```python
from build123d import *

# Parameters (mm, degrees)
SKETCH1_R           = 4
SKETCH1_R_2         = 5
BOSS_EXTRUDE1_DEPTH = 8
SKETCH2_R           = 7.75
CUT_EXTRUDE1_DEPTH  = 9


with BuildPart() as part:
    # Sketch1 → Boss-Extrude1 (new body)
    with BuildSketch(Plane.XY):
        Polygon((-55.929590299, 11.283196531), (55.49624814, 11.283196531), (55.49624814, -41.637870342), (-55.929590299, -41.637870342), (-55.929590299, -36.557898132), align=None)
        with Locations((38.28332892, -7.416803469)):
            Circle(SKETCH1_R, mode=Mode.SUBTRACT)
        with Locations((-0.21667108, -10.716803469)):
            Circle(SKETCH1_R_2, mode=Mode.SUBTRACT)
        with Locations((-38.71667108, -7.416803469)):
            Circle(SKETCH1_R, mode=Mode.SUBTRACT)
    extrude(amount=BOSS_EXTRUDE1_DEPTH)

    # Sketch2 → Cut-Extrude1 (cut, through all)
    with BuildSketch(Plane.XY.offset(8)):
        with Locations((-0.21667108, -10.716803469)):
            Circle(SKETCH2_R)
    extrude(amount=-CUT_EXTRUDE1_DEPTH, mode=Mode.SUBTRACT)


solid = part.part
```
Can you work these out from the model? Positions are in its coordinate system, mm. Coordinates: 2 decimals unless noted, no trailing zeros. Loops run counter-clockwise (first coordinate to the right, second up) from the corner with the lowest first, then second, coordinate; pieces in that order, holes last. Notation, with made-up numbers: M -33,81 L 21,81 A19 cw 21,87 Z; hole C 16.5,44 d2. An arc over 180 degrees is marked long. Put each result on its own line as item: value. Start each with the question number.
(1) Will this pin go through, and if not, where does the flat tip stop? pin 1 Ø5 at (x, y) = (-3, -14) entering from +Z.
(2) We'd pull the mould along X, two halves only. Please class faces 1 (the face through (-34.9, -6.22, 3.94)), 2 (the face through (-55.93, -15, 4)), 3 (the face through (1, -41.638, 4)): +X half, -X half, draft (parallel to the pull), parting line (faces both ways), or undercut.
(3) Imagine slicing it at A-A on x = -41.5. List the corners of the cut face in (y, z) for me, and give its area (3 significant figures).
(4) Imagine slicing it at C-C on y = -15. List the corners of the cut face in (x, z) for me, and give its area (3 significant figures).
(5) Imagine slicing it at B-B on z = 2.75. List the corners of the cut face in (x, y) for me.
(6) I need wall thicknesses on probe 1 along X at (y, z) = (-5.5, 6.75); probe 2 along X at (y, z) = (-8, 2.75); probe 3 along X at (y, z) = (-17, 7.75). Which ranges of each line are inside material? Lowest first, please.
Worked answers:
1. pin 1: passes through
2. face 1: undercut
2. face 2: -X half
2. face 3: draft
3. outline: M -41.64,0 L -10.29,0 L -10.29,8 L -41.64,8 Z; M -4.54,0 L 11.28,0 L 11.28,8 L -4.54,8 Z
3. area: 377 mm2
4. outline: M -55.93,0 L -6.68,0 L -6.68,8 L -55.93,8 Z; M 6.24,0 L 55.5,0 L 55.5,8 L 6.24,8 Z
4. area: 788 mm2
5. outline: M -55.93,-41.64 L 55.5,-41.64 L 55.5,11.28 L -55.93,11.28 Z; hole C -38.72,-7.42 d8; hole C -0.22,-10.72 d15.5; hole C 38.28,-7.42 d8
6. probe 1: x = -55.93 to -42.23, -35.21 to -5.95, 5.51 to 34.77, 41.79 to 55.5
6. probe 2: x = -55.93 to -42.67, -34.76 to -7.47, 7.04 to 34.33, 42.24 to 55.5
6. probe 3: x = -55.93 to -4.75, 4.32 to 55.5
